Can you work these out from the drawing? Everything is in mm from the part's minimum corner. A direction names the side the tool comes from. Give positions to 0.01 mm unless a question says otherwise; leave off trailing zeros. Write each loop counter-clockwise with the first axis right and the second up, starting at its lowest first coordinate (ties: lowest second). Pieces come first, ordered by that corner, then holes. Notation, with made-up numbers: M 15,-20 L 42,-20 A9 ccw 42,-16 Z; hole C 89.25,72 d2. An arc over 180 degrees is marked long. One line per item, written item: value.
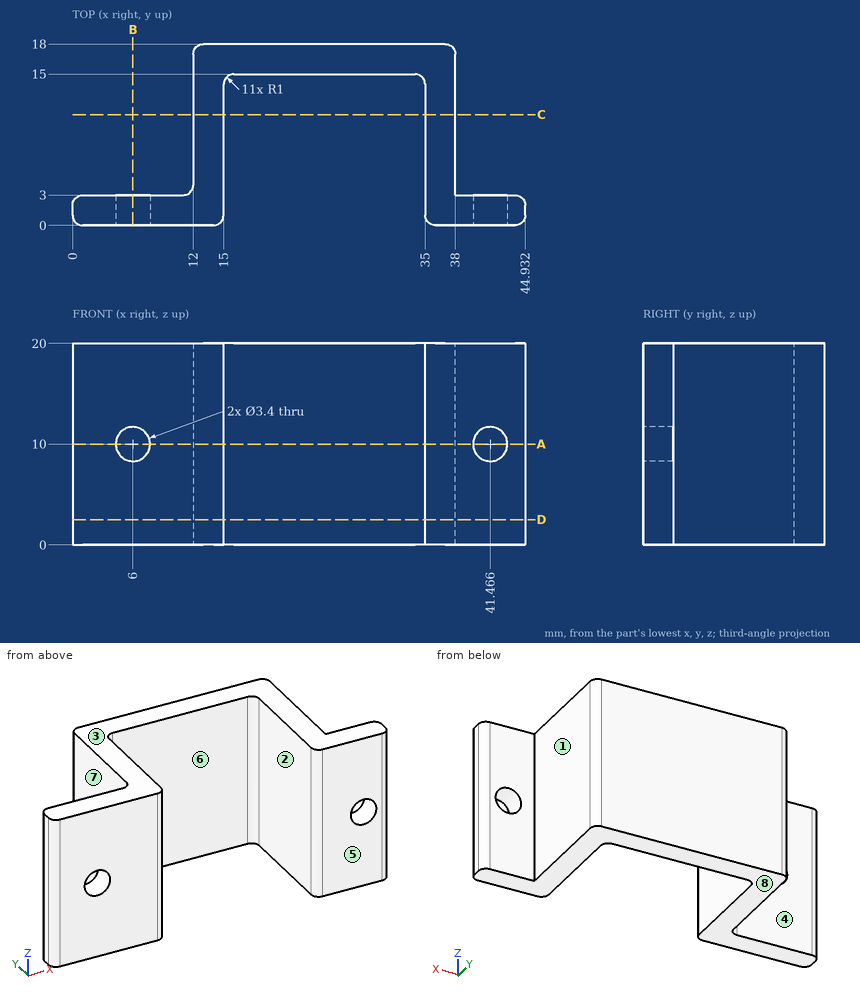
1) We'd pull the mould along X, two halves only. Please class the marked faces 6, 7 and 8: pulls with the +X half, pulls with the -X half, needs draft (parallel to the pull), parting line crosses it, or undercut.
Outcome:
face 6: undercut
face 7: pulls with the -X half
face 8: needs draft
2) Please list where these lines run through material, in increasing order: L1, parallel to X at y = 0.85, z = 10 (1 decimal); L2, parallel to X at y = 10, z = 8.5; L3, parallel to Z at x = 6, y = 1.15. Write a range as from..to.
Outcome:
L1: x = 0..4.3, 7.7..15, 35..39.8, 43.2..44.9
L2: x = 12..15, 35..38
L3: z = 0..8.3, 11.7..20
3) If we section it at A-A, the plane z = 10: Give the number of separate pieces and of enclosed holes in the cut face, then the cut area to 3 significant figures.
Outcome:
separate pieces: 3
enclosed holes: 0
area: 203 mm^2
4) If we section it at C-C, the plane y = 11: Write out the boundary of the cut face in (x, z), then the cut area to 3 significant figures.
Outcome:
outline: M 12,0 L 15,0 L 15,20 L 12,20 Z; M 35,0 L 38,0 L 38,20 L 35,20 Z
area: 120 mm^2
5) If we section it at D-D, the plane z = 2.5: Write out the boundary of the cut face in (x, y).
Outcome:
outline: M 0,1 A1 ccw 1,0 L 14,0 A1 ccw 15,1 L 15,14 A1 cw 16,15 L 34,15 A1 cw 35,14 L 35,1 A1 ccw 36,0 L 43.93,0 A1 ccw 44.93,1 L 44.93,2 A1 ccw 43.93,3 L 38,3 L 38,17 A1 ccw 37,18 L 13,18 A1 ccw 12,17 L 12,4 A1 cw 11,3 L 1,3 A1 ccw 0,2 Z
6) If we section it at B-B, the plane x = 6: Write out the boundary of the cut face in (y, z).
Outcome:
outline: M 0,0 L 3,0 L 3,8.3 L 0,8.3 Z; M 0,11.7 L 3,11.7 L 3,20 L 0,20 Z
7) On a 3-axis mill with a long thin cutter (end or side, diameter ignored), from which of +Z, -Z, +X, -X, +Y, -Y can I reach the whole of each face in a straight line? I mean the marked faces 1, 2, 3, 4 and 5. Say none if no direction works.
Outcome:
face 1: +Z, -Z, +X, +Y
face 2: +Z, -Z, -Y
face 3: +Z, +X, -X, +Y, -Y
face 4: +Z, -Z, -X, +Y
face 5: +Z, -Z, +X, -X, -Y
8) I'm going to push flat-ended pins straight in: pin 1 (4.5 mm diameter, centred on x = 42, z = 14.5, fed in from +Y); pin 2 (7 mm diameter, centred on y = 13, z = 14.5, fed in from +X); pin 3 (6 mm diameter, centred on y = 6.5, z = 10.5, fed in from -X). Where does each tip first touch, or does it pass through?
Outcome:
pin 1: stops at y = 3
pin 2: stops at x = 38
pin 3: stops at x = 11.87
